```python
from build123d import *

# Parameters (mm, degrees)
SKETCH1_R           = 2.5
BOSS_EXTRUDE1_DEPTH = 70
FILLET1_R           = 1
FILLET2_R           = 0.5
FILLET3_R           = 0.5
FILLET4_R           = 0.5
FILLET5_R           = 0.5


with BuildPart() as part:
    # Sketch1 → Boss-Extrude1 (new body)
    with BuildSketch(Plane.XY):
        Polygon((13.2, 0), (13.2, 1.8), (15.45, 1.8), (15.45, 3.6), (12.95, 6.1), (7.05, 6.1), (4.55, 3.6), (4.55, 1.8), (6.8, 1.8), (6.8, 0), (0, 0), (0, 6.8), (1.8, 6.8), (1.8, 4.55), (3.6, 4.55), (6.1, 7.05), (6.1, 12.95), (3.6, 15.45), (1.8, 15.45), (1.8, 13.2), (0, 13.2), (0, 20), (6.8, 20), (6.8, 18.2), (4.55, 18.2), (4.55, 16.4), (7.05, 13.9), (12.95, 13.9), (15.45, 16.4), (15.45, 18.2), (13.2, 18.2), (13.2, 20), (20, 20), (20, 13.2), (18.2, 13.2), (18.2, 15.45), (16.4, 15.45), (13.9, 12.95), (13.9, 7.05), (16.4, 4.55), (18.2, 4.55), (18.2, 6.8), (20, 6.8), (20, 0), align=None)
        with Locations((10, 10)):
            Circle(SKETCH1_R, mode=Mode.SUBTRACT)
    extrude(amount=BOSS_EXTRUDE1_DEPTH)

    # Fillet1
    fillet1_edges = [part.edges().sort_by_distance(p)[0] for p in [
        (0, 0, 35),
        (0, 20, 35),
        (20, 20, 35),
        (20, 0, 35),
    ]]
    fillet(fillet1_edges, radius=FILLET1_R)

    # Fillet2
    fillet2_edges = [part.edges().sort_by_distance(p)[0] for p in [
        (4.55, 18.2, 35),
        (4.55, 16.4, 35),
        (7.05, 13.9, 35),
        (12.95, 13.9, 35),
        (15.45, 16.4, 35),
        (15.45, 18.2, 35),
    ]]
    fillet(fillet2_edges, radius=FILLET2_R)

    # Fillet3
    fillet3_edges = [part.edges().sort_by_distance(p)[0] for p in [
        (18.2, 15.45, 35),
        (16.4, 15.45, 35),
        (13.9, 12.95, 35),
        (13.9, 7.05, 35),
        (16.4, 4.55, 35),
        (18.2, 4.55, 35),
    ]]
    fillet(fillet3_edges, radius=FILLET3_R)

    # Fillet4
    fillet4_edges = [part.edges().sort_by_distance(p)[0] for p in [
        (1.8, 4.55, 35),
        (3.6, 4.55, 35),
        (6.1, 7.05, 35),
        (6.1, 12.95, 35),
        (3.6, 15.45, 35),
        (1.8, 15.45, 35),
    ]]
    fillet(fillet4_edges, radius=FILLET4_R)

    # Fillet5
    fillet5_edges = [part.edges().sort_by_distance(p)[0] for p in [
        (15.45, 1.8, 35),
        (15.45, 3.6, 35),
        (12.95, 6.1, 35),
        (7.05, 6.1, 35),
        (4.55, 3.6, 35),
        (4.55, 1.8, 35),
    ]]
    fillet(fillet5_edges, radius=FILLET5_R)


solid = part.part
```
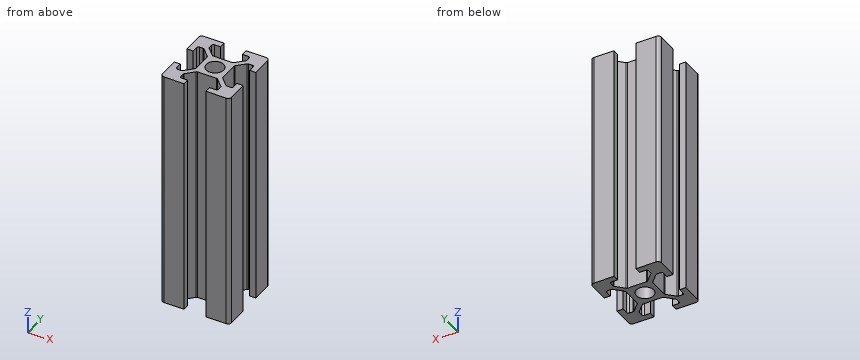
Geometry: final body of the model. Coordinates: model frame, mm. Coordinates: 2 decimals unless noted, no trailing zeros. Order: outer loops, then holes, each group sorted by start corner. A loop starts at its lowest first (then second) coordinate and runs counter-clockwise, first axis right, second up.
Item 1: Material intervals for line 1 along Y through (x, z) = (10, 51); line 2 along X through (y, z) = (2.25, 8); line 3 along X through (y, z) = (1, 26.5), sorted ascending.
Answer:
line 1: y = 6.1 to 7.5, 12.5 to 13.9
line 2: x = 0 to 4.55, 15.45 to 20
line 3: x = 0 to 6.8, 13.2 to 20
Item 2: Section query A-A (y = 10). Output: boundary loops of the cut face in (x, z), then the cut area to 3 significant figures.
Answer:
outline: (6.1, 0) - (7.5, 0) - (7.5, 70) - (6.1, 70) - close; (12.5, 0) - (13.9, 0) - (13.9, 70) - (12.5, 70) - close
area: 196 mm2
